Input: part model. Units: mm. Frame: model coordinates. Face numbers are marked on the shaded views. A direction names the side the tool comes from. Round coordinates to 2 decimals unless told otherwise and drop trailing zeros. Loops run counter-clockwise (first coordinate to the right, second up) from the corner with the lowest first, then second, coordinate; pieces in that order, holes last. Notation, with made-up numbers: (-1, 36.5) - (32, 36.5) arc R34 cw to (32, 75.5) - close; hole circle Ø8 at (-17.5, 2). An arc over 180 degrees is marked (long way). Write each question's results on one line, items separated by ' | '.
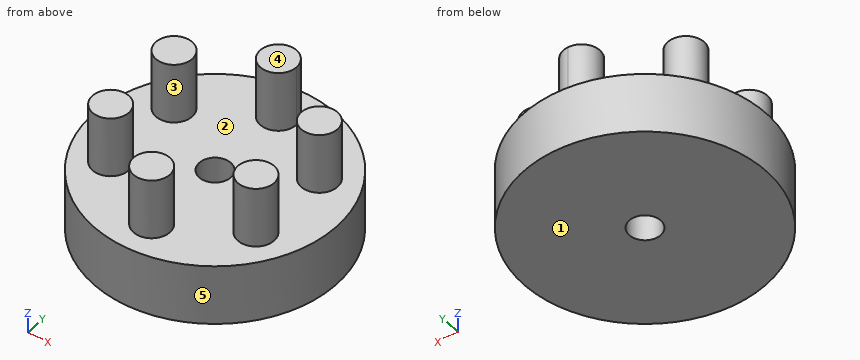
from build123d import *

# Parameters (mm, degrees)
F0_R     = 25.4
F0_R_2   = 3.302
F1_DEPTH = 12.7
F2_R     = 3.81
F3_DEPTH = 12.7


with BuildPart() as f1:
    # F0 (on Top) → F1 (new body)
    with BuildSketch(Plane.XY):
        Circle(F0_R)
        Circle(F0_R_2, mode=Mode.SUBTRACT)
    extrude(amount=F1_DEPTH)

    # F2 (on face) → F3 (join)
    with BuildSketch(Plane.XY.offset(12.7)):
        with BuildLine():
            ThreePointArc((0, 21.59), (-2.694077, 15.085923), (3.81, 17.78))
            ThreePointArc((3.81, 17.78), (2.694077, 20.474077), (0, 21.59))
        make_face()
        with Locations((-15.397932, 8.89)):
            Circle(F2_R)
        with Locations((-15.397932, -8.89)):
            Circle(F2_R)
        with Locations((0, -17.78)):
            Circle(F2_R)
        with Locations((15.397932, -8.89)):
            Circle(F2_R)
        with Locations((15.397932, 8.89)):
            Circle(F2_R)
    extrude(amount=F3_DEPTH)


solid = f1.part
1. Contact query for flat-ended pins moving along their axis: pin 1 (12 mm diameter, centred on x = 3.5, y = 8, fed in from +Z); pin 2 (3 mm diameter, centred on x = -8.5, z = 16.5, fed in from +Y); pin 3 (4 mm diameter, centred on y = 19.5, z = 11, fed in from +X); pin 4 (1.5 mm diameter, centred on y = 20, z = 16, fed in from +X) (3 decimals). Output: stop coordinate, or through.
Answer:
pin 1: z = 12.7 | pin 2: through | pin 3: x = 18.41 | pin 4: x = 3.515
2. Line query: line 1 (Y direction, x = 0, z = 3.75); line 2 (Z direction, x = 4, y = -11); line 3 (Y direction, x = 2.5, z = 7.75). Output: solid intervals per line, ascending. Write a range as [from, to].
Answer:
line 1: [-25.4, -3.3], [3.3, 25.4] | line 2: [0, 12.7] | line 3: [-25.28, -2.16], [2.16, 25.28]
3. Section query B-B, the plane y = 0. Output: boundary loops of the cut face in (x, z).
Answer:
outline: (-25.4, 0) - (-3.3, 0) - (-3.3, 12.7) - (-25.4, 12.7) - close; (3.3, 0) - (25.4, 0) - (25.4, 12.7) - (3.3, 12.7) - close
4. Section query A-A, the plane z = 17.5. Output: boundary loops of the cut face in (x, y).
Answer:
outline: circle Ø7.62 at (-15.4, -8.89); circle Ø7.62 at (-15.4, 8.89); circle Ø7.62 at (0, -17.78); circle Ø7.62 at (0, 17.78); circle Ø7.62 at (15.4, -8.89); circle Ø7.62 at (15.4, 8.89)
5. Mould query, pull axis X, two halves, no side actions, for the marked faces 3, 4 and 5. Classes: pulls with the +X half, pulls with the -X half, needs draft (parallel to the pull), parting line crosses it, or undercut.
Answer:
face 3: undercut | face 4: needs draft | face 5: parting line crosses it
6. Section query D-D, the plane z = 9. Output: boundary loops of the cut face in (x, y).
Answer:
outline: circle Ø50.8 at (0, 0); hole circle Ø6.6 at (0, 0)
7. Section query C-C, the plane y = -17.78. Output: boundary loops of the cut face in (x, z).
Answer:
outline: (-18.14, 0) - (18.14, 0) - (18.14, 12.7) - (3.81, 12.7) - (3.81, 25.4) - (-3.81, 25.4) - (-3.81, 12.7) - (-18.14, 12.7) - close
8. Set-up query: the marked faces 1 and 2. Return all of +Z, -Z, +X, -X, +Y, -Y with unobstructed straight access to the full face (end or side cutting, diameter ignored); none if empty.
Answer:
face 1: -Z, +X, -X, +Y, -Y | face 2: +Z
